Design review of the part built by this model. Coordinates are the model's own, in mm. Face numbers are marked on the shaded views. A direction names the side the tool comes from. Give positions to 0.01 mm unless a question says otherwise; leave off trailing zeros. Write each loop counter-clockwise with the first axis right and the second up, starting at its lowest first coordinate (ties: lowest second). Pieces come first, ordered by that corner, then holes. Notation, with made-up numbers: M -3.75,40.25 L 8.25,40.25 A28 cw 8.25,60.25 Z; hole C 7.25,-22 d11. An arc over 180 degrees is marked long. Answer in a Markdown table with one row per item.
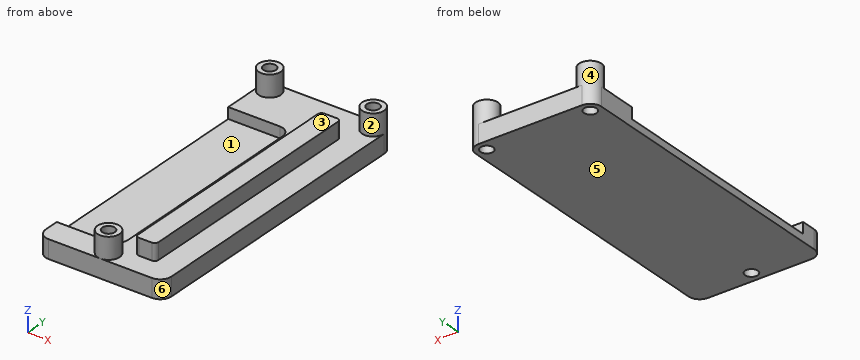
```python
from build123d import *

# Parameters (mm, degrees)
BOSS_EXTRU_2_DEPTH      = 5
ESQUISSE4_R             = 3
BOSS_EXTRU_3_DEPTH      = 5.8
D_GAGEMENT_M31_D        = 3.4
BOSS_EXTRU_4_DEPTH      = 4.5
ENL_V_MAT_EXTRU_1_DEPTH = 3


with BuildPart() as part:
    # Esquisse1 → Boss.-Extru.2 (new body)
    with BuildSketch(Plane.XY):
        with BuildLine():
            Line((3, 0), (31, 0))
            ThreePointArc((31, 0), (33.121320344, 0.878679656), (34, 3))
            Line((34, 3), (34, 80))
            ThreePointArc((34, 80), (33.121320344, 82.121320344), (31, 83))
            Line((31, 83), (3, 83))
            ThreePointArc((3, 83), (0.878679656, 82.121320344), (0, 80))
            Line((0, 80), (0, 3))
            ThreePointArc((0, 3), (0.878679656, 0.878679656), (3, 0))
        make_face()
    extrude(amount=BOSS_EXTRU_2_DEPTH)

    # Esquisse4 → Boss.-Extru.3 (add)
    with BuildSketch(Plane.XY.offset(5)):
        with Locations((3, 80)):
            Circle(ESQUISSE4_R)
        with Locations((31, 80)):
            Circle(ESQUISSE4_R)
        with Locations((17, 3)):
            Circle(ESQUISSE4_R)
    extrude(amount=BOSS_EXTRU_3_DEPTH)

    # Dégagement M31 (through all)
    with Locations(Plane.XY.offset(10.8)):
        with Locations((3, 80), (31, 80), (17, 3)):
            Hole(D_GAGEMENT_M31_D / 2)

    # Esquisse2 → Boss.-Extru.4 (add)
    with BuildSketch(Plane.XY.offset(5)):
        with BuildLine():
            Line((23, 73), (26.5, 73))
            ThreePointArc((26.5, 73), (27.207106781, 72.707106781), (27.5, 72))
            Line((27.5, 72), (27.5, 7))
            ThreePointArc((27.5, 7), (27.207106781, 6.292893219), (26.5, 6))
            Line((26.5, 6), (23, 6))
            ThreePointArc((23, 6), (22.292893219, 6.292893219), (22, 7))
            Line((22, 7), (22, 72))
            ThreePointArc((22, 72), (22.292893219, 72.707106781), (23, 73))
        make_face()
    extrude(amount=BOSS_EXTRU_4_DEPTH)

    # Esquisse7 → Enlèv. mat.-Extru.1 (cut)
    with BuildSketch(Plane.XY.offset(5)):
        with BuildLine():
            Line((14, 69), (0, 69))
            Line((0, 69), (0, 7))
            Line((0, 7), (14, 7))
            ThreePointArc((14, 7), (16.121320344, 7.878679656), (17, 10))
            Line((17, 10), (17, 66))
            ThreePointArc((17, 66), (16.121320344, 68.121320344), (14, 69))
        make_face()
    extrude(amount=-ENL_V_MAT_EXTRU_1_DEPTH, mode=Mode.SUBTRACT)


solid = part.part
```
1) Insertion check: P1, Ø4, axis at x = 17.5, y = 17.5, coming from the +Z side; P2, Ø2, axis at y = 49, z = 7, coming from the +X side; P3, Ø4.5, axis at x = 25, y = 28.5, coming from the +Z side. Each pin has a flat end and moves straight along its axis. Give the tip position at first contact, or say it passes through.
Geometry says:
| item | result |
|---|---|
| P1 | z = 5 |
| P2 | x = 27.5 |
| P3 | z = 9.5 |
2) For the marked faces 1, 2 and 3, list the 3-axis set-ups (+Z, -Z, +X, -X, +Y, -Y) from which the entire face can be reached by the end or side of a thin tool; tool diameter is ignored.
Geometry says:
| item | result |
|---|---|
| face 1 | +Z, -X |
| face 2 | +Z |
| face 3 | +Z, +X, -X, +Y, -Y |
3) Add section A-A (z = 7.5). Write out the cut boundary in (x, y), and give its area (3 significant figures).
Geometry says:
| item | result |
|---|---|
| outline | C 3,80 d6; C 17,3 d6; M 22,7 A1 ccw 23,6 L 26.5,6 A1 ccw 27.5,7 L 27.5,72 A1 ccw 26.5,73 L 23,73 A1 ccw 22,72 Z; C 31,80 d6; hole C 3,80 d3.4; hole C 17,3 d3.4; hole C 31,80 d3.4 |
| area | 425 mm^2 |
4) To check wall thickness, follow probe 1 along X at (y, z) = (80, 3.5); probe 2 along Y at (x, z) = (17, 7.5); probe 3 along Y at (x, z) = (8, 3). State the ranges of each line that lie inside material, in increasing order. Write a range as [from, to].
Geometry says:
| item | result |
|---|---|
| probe 1 | [0, 1.3], [4.7, 29.3], [32.7, 34] |
| probe 2 | [0, 1.3], [4.7, 6] |
| probe 3 | [0, 7], [69, 83] |
5) Add section B-B (z = 3.5). Write out the cut boundary in (x, y), and give its area (3 significant figures).
Geometry says:
| item | result |
|---|---|
| outline | M 0,3 A3 ccw 3,0 L 31,0 A3 ccw 34,3 L 34,80 A3 ccw 31,83 L 3,83 A3 ccw 0,80 L 0,69 L 14,69 A3 cw 17,66 L 17,10 A3 cw 14,7 L 0,7 Z; hole C 3,80 d3.4; hole C 17,3 d3.4; hole C 31,80 d3.4 |
| area | 1,740 mm^2 |
6) Add section C-C (y = 24.5). Write out the cut boundary in (x, z), and give its area (3 significant figures).
Geometry says:
| item | result |
|---|---|
| outline | M 0,0 L 34,0 L 34,5 L 27.5,5 L 27.5,9.5 L 22,9.5 L 22,5 L 17,5 L 17,2 L 0,2 Z |
| area | 144 mm^2 |
7) The part is to be moulded in two halves that separate along X. For the marked faces 4, 5 and 6, say which applies: released by +X, released by -X, zero draft, split by the parting line, or undercut.
Geometry says:
| item | result |
|---|---|
| face 4 | undercut |
| face 5 | zero draft |
| face 6 | released by +X |
